Design review of the part built by this model. Coordinates are the model's own, in mm. Round coordinates to 2 decimals unless told otherwise and drop trailing zeros. Loops run counter-clockwise (first coordinate to the right, second up) from the corner with the lowest first, then second, coordinate; pieces in that order, holes last. Notation, with made-up numbers: (-34.75, -22.75) -> (-19.75, -22.75) arc R18 cw to (-19.75, -0.75) -> close; hole circle Ø1 at (12, -28.75). An arc over 180 degrees is marked (long way). Answer as CSV lines item,"result". Start each with the question number.
(1) Take a section at B-B, the plane y = -339.5. Write out the cut boundary in (x, z).
(2) To check wall thickness, follow line 1 (X direction, y = -342.5, z = 3.4); line 2 (Y direction, x = -4, z = 4.55); line 3 (X direction, y = -12, z = 0.5). State the ranges of each line that lie inside material, in increasing order. Write a range as from..to.
(3) Take a section at C-C, the plane x = -59.5. Write out the cut boundary in (y, z), and give its area (3 significant figures).
(4) For P1, Ø1.5, axis at y = -370, z = 3, coming from the -X side; P2, Ø2.5, axis at x = -25.5, z = 2.5, coming from the +Y side; P3, Ø2.5, axis at y = -352.5, z = 2, coming from the -X side, all flat-tipped, find the tip position at first contact; note any pin that passes through.
(5) Take a section at D-D, the plane y = -104.5. Write out the cut boundary in (x, z).
(6) Take a section at A-A, the plane z = 1.15. Write out the cut boundary in (x, y), and give its area (3 significant figures).
from build123d import *

# Parameters (mm, degrees)
SKETCH_W  = 80
SKETCH_H  = 130
PAD_DEPTH = 5


with BuildPart() as part:
    # Sketch → Pad (new body)
    with BuildSketch(Plane.XY):
        with BuildLine():
            ThreePointArc((200, 3e-06), (141.421355, 141.421357), (0, 200))
            ThreePointArc((0, 200), (-141.421355, 141.421357), (-200, 3e-06))
            Line((-200, 3e-06), (-200, -347.34))
            ThreePointArc((-200, -347.34), (-169.931582, -419.931582), (-97.340001, -450))
            Line((0, -450), (-97.340001, -450))
            Line((0, -450), (97.340001, -450))
            ThreePointArc((97.340001, -450), (169.931582, -419.931582), (200, -347.34))
            Line((200, 3e-06), (200, -347.34))
        make_face()
        with BuildLine():
            Line((0, -300), (116, -300))
            Line((116, -300), (116, -250))
            Line((116, -250), (113, -250))
            Line((113, -250), (113, -0.000123))
            ThreePointArc((113, -0.000123), (79.90311, 79.903023), (0, 113))
            ThreePointArc((0, 113), (-79.90311, 79.903023), (-113, -0.000123))
            Line((-113, -250), (-113, -0.000123))
            Line((-116, -250), (-113, -250))
            Line((-116, -300), (-116, -250))
            Line((0, -300), (-116, -300))
        make_face(mode=Mode.SUBTRACT)
        with Locations((80, -375)):
            Rectangle(SKETCH_W, SKETCH_H, mode=Mode.SUBTRACT)
        Polygon((0, -310), (30, -310), (30, -440), (0, -440), (-30, -440), (-30, -310), align=None, mode=Mode.SUBTRACT)
        with Locations((-80, -375)):
            Rectangle(SKETCH_W, SKETCH_H, mode=Mode.SUBTRACT)
    extrude(amount=PAD_DEPTH)


solid = part.part
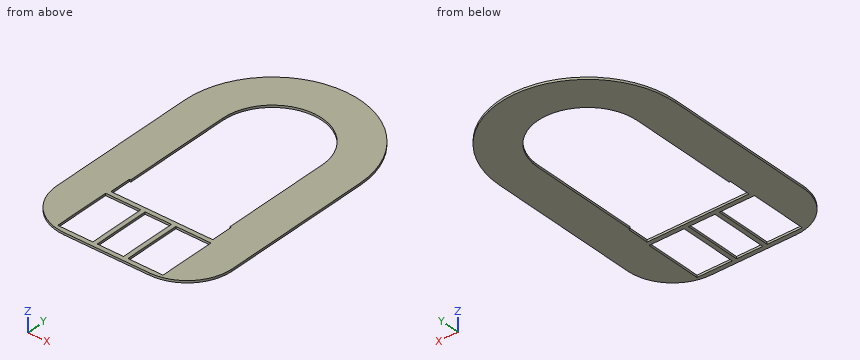
The answers:
1,outline,"(-200, 0) -> (-120, 0) -> (-120, 5) -> (-200, 5) -> close; (-40, 0) -> (-30, 0) -> (-30, 5) -> (-40, 5) -> close; (30, 0) -> (40, 0) -> (40, 5) -> (30, 5) -> close; (120, 0) -> (200, 0) -> (200, 5) -> (120, 5) -> close"
2,line 1,"-200..-120, -40..-30, 30..40, 120..200"
2,line 2,"-450..-440, -310..-300, 112.93..199.96"
2,line 3,"-200..-113, 113..200"
3,outline,"(-450, 0) -> (-440, 0) -> (-440, 5) -> (-450, 5) -> close; (-310, 0) -> (-300, 0) -> (-300, 5) -> (-310, 5) -> close; (96.07, 0) -> (190.94, 0) -> (190.94, 5) -> (96.07, 5) -> close"
3,area,"574 mm²"
4,P1,"x = -197.63"
4,P2,"y = 198.52"
4,P3,"x = -199.93"
5,outline,"(-200, 0) -> (-113, 0) -> (-113, 5) -> (-200, 5) -> close; (113, 0) -> (200, 0) -> (200, 5) -> (113, 5) -> close"
6,outline,"(-200, -347.34) arc R102.66 ccw to (-97.34, -450) -> (97.34, -450) arc R102.66 ccw to (200, -347.34) -> (200, 0) arc R200 ccw to (0, 200) arc R200 ccw to (-200, 0) -> close; hole (-120, -440) -> (-40, -440) -> (-40, -310) -> (-120, -310) -> close; hole (-116, -300) -> (116, -300) -> (116, -250) -> (113, -250) -> (113, 0) arc R113 ccw to (0, 113) arc R113 ccw to (-113, 0) -> (-113, -250) -> (-116, -250) -> close; hole (-30, -440) -> (30, -440) -> (30, -310) -> (-30, -310) -> close; hole (40, -440) -> (120, -440) -> (120, -310) -> (40, -310) -> close"
6,area,"122,000 mm²"
